Work out the finished part from the listing and answer in its coordinate system (mm). A direction names the side the tool comes from. Round coordinates to 2 decimals unless told otherwise and drop trailing zeros. Order: outer loops, then holes, each group sorted by start corner. A loop starts at its lowest first (then second) coordinate and runs counter-clockwise, first axis right, second up. Notation, with made-up numbers: (88.25, 89) - (117.25, 89) arc R35 cw to (117.25, 123) - close; hole circle Ø3 at (41.25, 82.25). An arc over 180 degrees is marked (long way). One line per question, with ' | ' between items. Start each with the question number.
from build123d import *

# Parameters (mm, degrees)
SKETCH_W          = 35.3624
SKETCH_H          = 77.7328
PAD_DEPTH         = 8.5
PAD_DEPTH_BACK    = 6
SKETCH002_W       = 30.3624
SKETCH002_H       = 72.7328
POCKET_DEPTH      = 3.5
POCKET_DEPTH_BACK = 8.5
SKETCH003_W       = 5
SKETCH003_H       = 5
PAD001_DEPTH      = 8.5
PAD001_DEPTH_BACK = 3.5
SKETCH004_W       = 5.1844
SKETCH004_H       = 5.1948
SKETCH004_H_2     = 5
PAD002_DEPTH      = 3.5
SKETCH005_W       = 5.1844
SKETCH005_H       = 2.5
PAD003_DEPTH      = 1.6
PAD003_DEPTH_BACK = 3.5
SKETCH006_R       = 1.15
POCKET001_DEPTH   = 8
SKETCH007_R       = 4.5
POCKET002_DEPTH   = 2.5
POCKET003_DEPTH   = 2.5


with BuildPart() as part:
    # Sketch → Pad (new body, two sides)
    with BuildSketch(Plane.XY) as pad_sk:
        with Locations((14.6812, 25.8664)):
            Rectangle(SKETCH_W, SKETCH_H)
    extrude(amount=PAD_DEPTH)
    extrude(pad_sk.sketch, amount=-PAD_DEPTH_BACK)

    # Sketch002 → Pocket (cut, two sides)
    with BuildSketch(Plane.XY) as pocket_sk:
        with Locations((14.6812, 25.8664)):
            Rectangle(SKETCH002_W, SKETCH002_H)
    extrude(amount=-POCKET_DEPTH, mode=Mode.SUBTRACT)
    extrude(pocket_sk.sketch, amount=POCKET_DEPTH_BACK, mode=Mode.SUBTRACT)

    # Sketch003 → Pad001 (join, two sides)
    with BuildSketch(Plane.XY) as pad001_sk:
        with Locations((29.8624, -10.5)):
            Rectangle(SKETCH003_W, SKETCH003_H)
        with Locations((-0.5, -10.5)):
            Rectangle(SKETCH003_W, SKETCH003_H)
        with Locations((-0.5, 62.2328)):
            Rectangle(SKETCH003_W, SKETCH003_H)
        with Locations((29.8624, 62.2328)):
            Rectangle(SKETCH003_W, SKETCH003_H)
    extrude(amount=PAD001_DEPTH)
    extrude(pad001_sk.sketch, amount=-PAD001_DEPTH_BACK)

    # Sketch004 → Pad002 (join)
    with BuildSketch(Plane.XY):
        with Locations((2.0922, 57.1354)):
            Rectangle(SKETCH004_W, SKETCH004_H)
        with Locations((27.2702, 57.1354)):
            Rectangle(SKETCH004_W, SKETCH004_H)
        with Locations((2.0922, 2.174)):
            Rectangle(SKETCH004_W, SKETCH004_H_2)
        with Locations((27.2702, 2.174)):
            Rectangle(SKETCH004_W, SKETCH004_H_2)
    extrude(amount=-PAD002_DEPTH)

    # Sketch005 → Pad003 (join, two sides)
    with BuildSketch(Plane.XY) as pad003_sk:
        with Locations((27.2702, -1.576)):
            Rectangle(SKETCH005_W, SKETCH005_H)
        with Locations((2.0922, -1.576)):
            Rectangle(SKETCH005_W, SKETCH005_H)
    extrude(amount=PAD003_DEPTH)
    extrude(pad003_sk.sketch, amount=-PAD003_DEPTH_BACK)

    # Sketch006 (on DatumPlane) → Pocket001 (cut)
    with BuildSketch(Plane.XY.offset(8.5)):
        with Locations((29.8624, -10.5)):
            Circle(SKETCH006_R)
        with Locations((-0.5, -10.5)):
            Circle(SKETCH006_R)
        with Locations((29.8624, 62.2328)):
            Circle(SKETCH006_R)
        with Locations((-0.5, 62.2328)):
            Circle(SKETCH006_R)
    extrude(amount=-POCKET001_DEPTH, mode=Mode.SUBTRACT)

    # Sketch007 (on DatumPlane) → Pocket002 (cut)
    with BuildSketch(Plane.XZ.offset(13)):
        with Locations((9, 2.5)):
            Circle(SKETCH007_R)
    extrude(amount=-POCKET002_DEPTH, mode=Mode.SUBTRACT)

    # Sketch008 (on DatumPlane) → Pocket003 (cut)
    with BuildSketch(Plane(origin=(-3, 0, 0), x_dir=(0, -1, 0), z_dir=(-1, 0, 0))):
        Polygon((-47.9278, 2.85), (-43.4528, 2.85), (-43.4528, 4.35), (-39.4528, 4.35), (-39.4528, 2.85), (-34.9778, 2.85), (-34.9778, 1.35), (-39.4528, 1.35), (-39.4528, -0.15), (-43.4528, -0.15), (-43.4528, 1.35), (-47.9278, 1.35), align=None)
    extrude(amount=-POCKET003_DEPTH, mode=Mode.SUBTRACT)


solid = part.part
1) Straight lines are drawn through the part: line 1 (Y direction, x = 21, z = 7.75); line 2 (X direction, y = 19, z = -3); line 3 (Y direction, x = 0.5, z = 2.25). For each, find the intervals that lie inside material, in ascending order.
2) For faces 5 (the flat face through (-2, 34.978, 2)), 6 (the flat face through (24.678, 57, -2)), determine the directions among +Z, -Z, +X, -X, +Y, -Y from which every point of the face is accessible in a straight line to the end or side of a thin tool.
3) Section A-A on x = 9 is taken. Give the vertices of the cut face in (y, z).
4) Section C-C on x = 20.5 is taken. Give the vertices of the cut face in (y, z), and give its area (3 significant figures).
5) Determine the mould class of faces 1 (the cylindrical face through (-0.749, -11.623, 4.556)), 2 (the flat face through (14, 64.733, 1)), 3 (the flat face through (32.362, 25, 1)), 4 (the flat face through (-2, 41, 4.35)) for opening direction Y: released by +Y, released by -Y, zero draft, split by the parting line, or undercut.
6) Flat-ended cylindrical pins translate along their axes: pin 1 (9 mm diameter, centred on x = 13.5, y = 30.5, fed in from +Z); pin 2 (4 mm diameter, centred on x = 26.5, y = 57.5, fed in from +Z); pin 3 (3 mm diameter, centred on x = 26, y = -1.5, fed in from +Z). Find the tip coordinate at first contact, or state that the pin passes through.
7) Section D-D on z = 5.25 is taken. Give the vertices of the cut face in (x, y).
8) Section B-B on y = -5 is taken. Give the vertices of the cut face in (x, z).
Recorded:
1) line 1: y = -13 to -10.5, 62.23 to 64.73 | line 2: x = -3 to -0.5, 29.86 to 32.36 | line 3: y = -13 to -11.07, -9.93 to -8, 59.73 to 61.66, 62.8 to 64.73
2) face 5: -X | face 6: +Z
3) outline: (-13, -6) - (64.73, -6) - (64.73, 8.5) - (62.23, 8.5) - (62.23, -3.5) - (-10.5, -3.5) - (-10.5, -2) - (-13, -2) - close; (-13, 7) - (-10.5, 7) - (-10.5, 8.5) - (-13, 8.5) - close
4) outline: (-13, -6) - (64.73, -6) - (64.73, 8.5) - (62.23, 8.5) - (62.23, -3.5) - (-10.5, -3.5) - (-10.5, 8.5) - (-13, 8.5) - close | area: 254 mm²
5) face 1: undercut | face 2: released by +Y | face 3: zero draft | face 4: undercut
6) pin 1: stops at z = -3.5 | pin 2: stops at z = 0 | pin 3: stops at z = 1.6
7) outline: (-3, -13) - (5.44, -13) - (5.44, -10.5) - (2, -10.5) - (2, -8) - (-0.5, -8) - (-0.5, 59.73) - (2, 59.73) - (2, 62.23) - (27.36, 62.23) - (27.36, 59.73) - (29.86, 59.73) - (29.86, -8) - (27.36, -8) - (27.36, -10.5) - (12.56, -10.5) - (12.56, -13) - (32.36, -13) - (32.36, 64.73) - (-3, 64.73) - close; hole circle Ø2.3 at (-0.5, -10.5); hole circle Ø2.3 at (-0.5, 62.23); hole circle Ø2.3 at (29.86, -10.5); hole circle Ø2.3 at (29.86, 62.23)
8) outline: (-3, -6) - (32.36, -6) - (32.36, 8.5) - (29.86, 8.5) - (29.86, -3.5) - (-0.5, -3.5) - (-0.5, 8.5) - (-3, 8.5) - close
